Read the model definition and answer for the solid it produces. Units are mm, in the model's axes. Face numbers are marked on the shaded views. A direction names the side the tool comes from. Coordinates: 2 decimals unless noted, no trailing zeros. Loops run counter-clockwise (first coordinate to the right, second up) from the corner with the lowest first, then second, coordinate; pieces in that order, holes last.
Q1. The mould has two halves that part along Z. Classify the marked faces 4, 5, 6 and 7: pulls with the +Z half, pulls with the -Z half, needs draft (parallel to the pull), parting line crosses it, or undercut.
Q2. Flat-ended cylindrical pins translate along their axes: P1, Ø5, axis at x = -131, z = 6, coming from the -Y side; P2, Ø1, axis at x = -85.5, z = -53, coming from the -Y side; P3, Ø6, axis at y = -41.5, z = -60, coming from the -X side; P4, Ø22.5, axis at x = -81.5, y = -63, coming from the -Z side. Find the tip coordinate at first contact, or state that the pin passes through.
Q3. Section C-C (x = -93) is taken. Give the vertices of the cut face in (y, z) (1 decimal), then the cut area to 3 significant figures.
Q4. Section B-B (z = -23) is taken. Give the vertices of the cut face in (x, y) (3 decimals).
Q5. Section A-A (x = -58) is taken. Give the vertices of the cut face in (y, z) (1 decimal).
Q6. Straight lines are drawn through the part: line 1 (Z direction, x = -66, y = -35); line 2 (Z direction, x = -52, y = -3.5); line 3 (X direction, y = -34.5, z = -54). For each, find the intervals that lie inside material, in ascending order.
Q7. Which of the six approach directions +Z, -Z, +X, -X, +Y, -Y give full straight-line access (tool end or side, diameter ignored) to the marked faces 1, 2 and 3?
Autodesk Inventor part; units mm, degrees
ref_plane "YZ Plane" through (0, 0, 0) normal (1, 0, 0) x (0, 1, 0)
ref_plane "XZ Plane" through (0, 0, 0) normal (0, 1, 0) x (-1, 0, 0)
ref_plane "XY Plane" through (0, 0, 0) normal (0, 0, 1) x (1, 0, 0)
sketch "Sketch3" plane through (0, 0, 0) normal (1, 0, 0) x (0, 1, 0)
  line L0 (-85.725, 0) -> (-85.725, -1.5875)
  line L1 (-85.725, -1.5875) -> (-85.725, 1.5875)
  line L2 (-85.725, 1.5875) -> (-9.3918, 1.5875)
  line L3 (-85.725, -1.5875) -> (-9.3918, -1.5875)
  line L4 (-85.725, -50.8) -> (-85.725, -49.2125)
  line L5 (-85.725, -49.2125) -> (-85.725, -52.3875)
  line L6 (-85.725, -52.3875) -> (-9.3918, -52.3875)
  line L7 (-85.725, -49.2125) -> (-9.3918, -49.2125)
  circle A0 centre (0, 0) radius 9.525
  circle A1 centre (0, -50.8) radius 9.525
  line L8 (-98.425, 1.5875) -> (12.7, 12.7)
  line L9 (-98.425, -52.3875) -> (12.7, -63.5)
  line L10 (12.7, 12.7) -> (12.7, -63.5)
  line L11 (-98.425, -52.3875) -> (-98.425, 1.5875)
  line L12 (19.05, -70.5167) -> (-104.775, -58.1342)
  line L13 (-104.775, -58.1342) -> (-104.775, 7.3342)
  line L14 (-104.775, 7.3342) -> (19.05, 19.7167)
  line L15 (19.05, 19.7167) -> (19.05, -70.5167)
  dimension "d14" = 1.5875
  dimension "d15" = 3.175
  dimension "d40" = 6.35
extrude "Extrusion2" add sketch "Sketch3" along normal blind 12.7 contours L1 L2 A0 L3 L0 | A0 | L4 L7 A1 L6 L5 | A1 | L8 L10 L9 L11 | L12 L13 L14 L15
extrude "Extrusion3" add sketch "Sketch3" against normal blind 152.4 contours A0 | A1
extrude "Extrusion4" add sketch "Sketch3" against normal blind 127 contours L1 L2 A0 L3 L0 | L4 L7 A1 L6 L5
sketch "Sketch4" plane through (-127, -9.3918, 1.5875) normal (0, 0, 1) x (1, 0, 0)
  line L0 (0, -0.1332) -> (-25.4, -0.1332)
  line L1 (127, -76.3332) -> (0, -76.3332)
  line L2 (0, -0.1332) -> (127, -76.3332)
  line L3 (127, -76.3332) -> (0, -76.3332)
  line L4 (0, 0) -> (0, -0.1332)
  line L5 (0, -76.3332) -> (0, -0.1332)
  point P0 (127, 9.3918)
extrude "Extrusion5" cut sketch "Sketch4" against normal blind 127
draft "FaceDraft2" angle 0.4 pull direction (-1, 0, 0) faces at (-93.1333, -8.9299, 3.314) fixed edges at (-127, -9.4916, -0.7965) (-127, -9.4916, 0.7965)
draft "FaceDraft3" angle 0.4 pull direction (-1, 0, 0) faces at (-93.1333, -8.9299, -47.486) fixed edges at (-127, -9.4916, -51.5965) (-127, -9.4916, -50.0035)
fillet "Fillet3" radius 6.35 2 edges at (-152.4, -9.3477, 0) (-152.4, -9.3477, -50.8)
fillet "Fillet5" radius 6.35 4 edges at (6.35, 19.05, -70.5167) (6.35, 19.05, 19.7167) (6.35, -104.775, -58.1342) (6.35, -104.775, 7.3342)
fillet "Fillet6" radius 3.175 9 edges at (0, -103.1332, 5.8484) (0, -104.775, -25.4) (0, -103.1332, -56.6484) (0, -36.8284, -64.9288) (0, -92.3909, -59.3726) (0, 16.9609, -68.2082) (0, 19.05, -25.4) (0, 16.9609, 17.4082) (0, -43.4943, 13.4622)
chamfer "Chamfer1" distance 1.0583 angle 45 8 edges at (0, 0.7961, -40.4188) (0, 0.7961, -61.1812) (0, -48.0075, -52.3875) (0, 0.7961, 10.3812) (0, 0.7961, -10.3812) (0, -48.0075, -1.5875) (0, -48.0075, -49.2125) (0, -48.0075, 1.5875)
properties part number "Ski Rack"
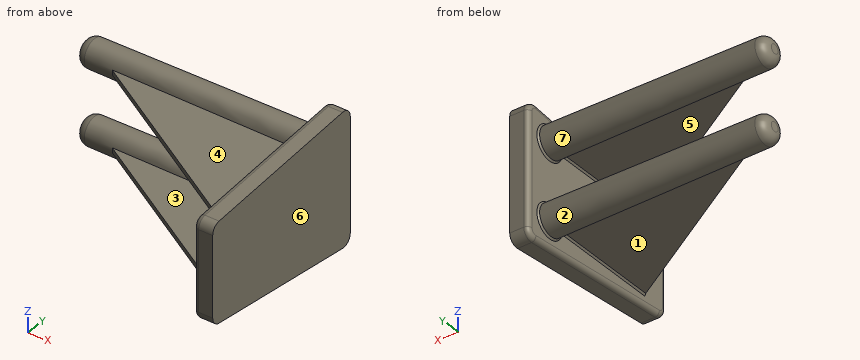
Numbers:
1. face 4: pulls with the +Z half
1. face 5: undercut
1. face 6: needs draft
1. face 7: undercut
2. P1: stops at y = -8.83
2. P2: stops at y = -9.67
2. P3: stops at x = 0
2. P4: passes through
3. outline: (-29.9, -52.4) - (-9.6, -52.4) arc R9.8 ccw (long way) to (-9.6, -49.2) - (-29.9, -49.2) - close; (-29.9, -1.6) - (-9.6, -1.6) arc R9.8 ccw (long way) to (-9.6, 1.6) - (-29.9, 1.6) - close
3. area: 727 mm2
4. outline: (0, -101.6) arc R3.175 ccw to (3.175, -104.775) - (12.7, -104.775) - (12.7, 19.05) - (3.175, 19.05) arc R3.175 ccw to (0, 15.875) - close
5. outline: (-50.9, -52.4) - (-9.9, -52.4) arc R10 ccw (long way) to (-9.9, -49.2) - (-50.9, -49.2) - close; (-50.9, -1.6) - (-9.9, -1.6) arc R10 ccw (long way) to (-9.9, 1.6) - (-50.9, 1.6) - close
6. line 1: z = -52.39 to -49.21, -1.59 to 1.59
6. line 2: z = -60.22 to -41.38, -9.42 to 9.42
6. line 3: x = 0 to 12.7
7. face 1: -Z, -X, -Y
7. face 2: -X
7. face 3: -X, -Y
